from build123d import *
from build123d.topology import SkipClean

# Parameters (mm, degrees)
ESBO_O1_R                = 6
RESSALTO_EXTRUS_O1_DEPTH = 5
RESSALTO_EXTRUS_O2_DEPTH = 24
ESBO_O3_R                = 2
RESSALTO_EXTRUS_O3_DEPTH = 6
ESBO_O5_R                = 15
CORTE_EXTRUS_O1_DEPTH    = 10


with BuildPart() as part:
    # Esboço1 → Ressalto-extrusão1 (new body)
    with BuildSketch(Plane.XY):
        with BuildLine():
            Line((-12, 0), (-12, 17))
            Line((-12, 17), (12, 17))
            Line((12, 17), (12, 0))
            ThreePointArc((12, 0), (0, -12), (-12, 0))
        make_face()
        Circle(ESBO_O1_R, mode=Mode.SUBTRACT)
    extrude(amount=RESSALTO_EXTRUS_O1_DEPTH)

    # Esboço2 → Ressalto-extrusão2 (add)
    with BuildSketch(Plane.ZY.offset(12)):
        Polygon((5, 17), (0.2, 17), (-10.8, 17), (-16.8, 17), (-16.8, 52), (11.2, 52), (11.2, 44), (5, 44), (5, 41.5), (8.3, 41.5), (5.3, 38.5), (-2.5, 38.5), (-5.5, 41.5), (-2.5, 41.5), (-2.5, 44), (-10.8, 44), (-10.8, 23), (-2.5, 23), (-2.5, 25), (-5.5, 25), (-2.5, 28), (5.3, 28), (8.3, 25), (5, 25), align=None)
    extrude(amount=-RESSALTO_EXTRUS_O2_DEPTH)

    # Esboço3 → Ressalto-extrusão3 (add)
    with BuildSketch(Plane(origin=(0, 52, 0), x_dir=(1, 0, 0), z_dir=(0, 1, 0))):
        with BuildLine():
            Line((12, -6), (-12, -6))
            Line((-12, -6), (-12, 2))
            Line((-12, 2), (-24, -6))
            Line((-24, -6), (-24, -12.72))
            Line((-24, -12.72), (-12, -12.72))
            ThreePointArc((-12, -12.72), (0, -6.72), (12, -12.72))
            Line((12, -12.72), (24, -12.72))
            Line((24, -12.72), (24, -6))
            Line((24, -6), (12, 2))
            Line((12, 2), (12, -6))
        make_face()
        with Locations(Location((19, -9.36, 0), (0, 0, 90))):
            Circle(ESBO_O3_R, mode=Mode.SUBTRACT)
        with Locations(Location((-19, -9.36, 0), (0, 0, 90))):
            Circle(ESBO_O3_R, mode=Mode.SUBTRACT)
    extrude(amount=-RESSALTO_EXTRUS_O3_DEPTH)

    # Esboço5 → Corte-extrusão1 (cut)
    with SkipClean():  # the faces are left unmerged after this step: merging them gives an invalid solid
        with BuildSketch(Plane(origin=(0, 52, 0), x_dir=(1, 0, 0), z_dir=(0, 1, 0))):
            with Locations((0, -21.72)):
                Circle(ESBO_O5_R)
        extrude(amount=-CORTE_EXTRUS_O1_DEPTH, mode=Mode.SUBTRACT)


solid = part.part
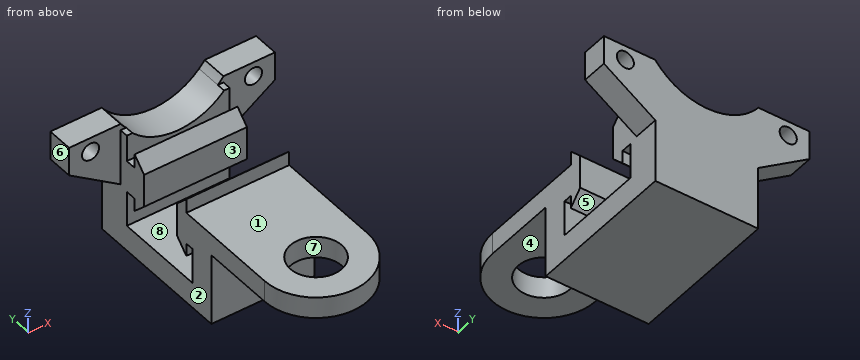
Work out the finished part from the listing and answer in its coordinate system (mm). Face numbers are marked on the shaded views. A direction names the side the tool comes from. Coordinates: 2 decimals unless noted, no trailing zeros. Write each loop counter-clockwise with the first axis right and the second up, starting at its lowest first coordinate (ties: lowest second). Pieces come first, ordered by that corner, then holes. Notation, with made-up numbers: (45.25, 80.25) - (53.25, 80.25) arc R30 cw to (53.25, 119.25) - close; hole circle Ø2 at (18.25, 35.5). An arc over 180 degrees is marked (long way). One line per question, with ' | ' between items.
1) For the marked faces 1, 2, 3, 4 and 5, determine the directions among +Z, -Z, +X, -X, +Y, -Y from which every point of the face is accessible in a straight line to the end or side of a thin tool.
Checks:
face 1: +Z, +X, -X, -Y | face 2: -Z, -X, -Y | face 3: +Z, +X, -X | face 4: -Z, +X, -X, -Y | face 5: +X, -X
2) Find section B-B, the plane z = -3.5. Determine the outline of the cut face in (x, y).
Checks:
outline: (-12, 17) - (12, 17) - (12, 23) - (-12, 23) - close; (-12, 25) - (12, 25) - (12, 27) - (-12, 27) - close; (-12, 39.5) - (12, 39.5) - (12, 41.5) - (-12, 41.5) - close; (-12, 44) - (12, 44) - (12, 52) - (-12, 52) - close
3) Flat-ended cylindrical pins translate along their axes: P1, Ø0.8, axis at x = -2, y = 42.5, coming from the +Z side; P2, Ø12, axis at y = 0, z = -11, coming from the +X side; P3, Ø3.5, axis at x = -3.5, z = 7, coming from the -Y side; P4, Ø6.5, axis at x = 19, z = 9.36, coming from the +Y side. Find the tip coordinate at first contact, or state that the pin passes through.
Checks:
P1: z = 5 | P2: through | P3: y = 25 | P4: y = 52
4) Find section D-D, the plane y = -1.5. Determine the outline of the cut face in (x, z), and give its area (3 significant figures).
Checks:
outline: (-11.91, 0) - (-5.81, 0) - (-5.81, 5) - (-11.91, 5) - close; (5.81, 0) - (11.91, 0) - (11.91, 5) - (5.81, 5) - close | area: 61.0 mm2
5) Find section C-C, the plane y = 39.5. Determine the outline of the cut face in (x, z), and give its area (3 significant figures).
Checks:
outline: (-12, -16.8) - (12, -16.8) - (12, -10.8) - (-12, -10.8) - close; (-12, -3.5) - (12, -3.5) - (12, 6.3) - (-12, 6.3) - close | area: 379 mm2
6) The mould has two halves that part along X. Classify the marked faces 6, 7 and 8: +X half, -X half, draft (parallel to the pull), parting line (faces both ways), or undercut.
Checks:
face 6: -X half | face 7: undercut | face 8: draft
7) Consider probe 1 along X at (y, z) = (47.4, 9.36); probe 2 along Y at (x, z) = (9, -3.5); probe 3 along Y at (x, z) = (-2.5, -0.75). Determine where each line is inside the solid, lowest interval first. Write a range as [from, to].
Checks:
probe 1: [-24, -21], [-17, -8.5], [8.5, 17], [21, 24] | probe 2: [17, 23], [25, 27], [39.5, 41.5], [44, 52] | probe 3: [17, 28], [38.5, 52]
8) Find section A-A, the plane x = 0. Determine the outline of the cut face in (y, z), and give its area (3 significant figures).
Checks:
outline: (-12, 0) - (-6, 0) - (-6, 5) - (-12, 5) - close; (6, 0) - (17, 0) - (17, -16.8) - (52, -16.8) - (52, 6.72) - (44, 6.72) - (44, 5) - (41.5, 5) - (41.5, 8.3) - (38.5, 5.3) - (38.5, -2.5) - (41.5, -5.5) - (41.5, -2.5) - (44, -2.5) - (44, -10.8) - (23, -10.8) - (23, -2.5) - (25, -2.5) - (25, -5.5) - (28, -2.5) - (28, 5.3) - (25, 8.3) - (25, 5) - (6, 5) - close | area: 629 mm2
